from build123d import *

# Parameters (mm, degrees)
F0_W     = 60.565564
F0_H     = 97.339354
F1_DEPTH = 2.286
F2_R     = 2.032
F3_W     = 7.62
F3_H     = 3.81
F4_DEPTH = 0.127


with BuildPart() as f1:
    # F0 (on Front) → F1 (new body)
    with BuildSketch(Plane.XZ):
        Rectangle(F0_W, F0_H)
    extrude(amount=F1_DEPTH)

    # F2
    f2_edges = [f1.edges().sort_by_distance(p)[0] for p in [
        (30.282782, -2.286, 0),
        (-30.282782, -2.286, 0),
    ]]
    fillet(f2_edges, radius=F2_R)

    # F3 (on face) → F4 (join, symmetric)
    with BuildSketch(Plane(origin=(0, 0, 0), x_dir=(-1, 0, 0), z_dir=(0, 1, 0))):
        with Locations((-26.472782, -46.764677)):
            Rectangle(F3_W, F3_H)
        with Locations((26.472782, -46.764677)):
            Rectangle(F3_W, F3_H)
    extrude(amount=F4_DEPTH, both=True)


solid = f1.part
Could you check a few things on this model? Use its own coordinates, in mm. Give positions to 0.01 mm unless a question says otherwise; leave off trailing zeros. Write each loop counter-clockwise with the first axis right and the second up, starting at its lowest first coordinate (ties: lowest second). Pieces come first, ordered by that corner, then holes. Notation, with made-up numbers: (43, -15) - (99, -15) arc R22 cw to (99, 13) - close; hole circle Ø3 at (17, 23.5). An arc over 180 degrees is marked (long way). Use CSV: the item, a comma, the result in double quotes. Start each with the question number.
Item 1: I want a section at B-B, the plane x = -1. Please give me the cut outline in (y, z), then the cut area to 3 significant figures.
Item 2: I'm going to push a flat-ended pin straight in: pin 1 (18 mm diameter, centred on x = -14, z = -3.5, fed in from +Y). Where does the tip first touch, or does it pass through?
Item 3: If I drill on line 1 along Y through (x, z) = (18, -6.5); line 2 along X through (y, z) = (-0.35, -29); line 3 along X through (y, z) = (-1.7, -43), over which ranges is the centre line in solid material (lowest first)?
Item 4: I want a section at A-A, the plane z = 6. Please give me the cut outline in (x, y), then the cut area to 3 significant figures.
Item 5: I want a section at C-C, the plane y = -1.6. Please give me the cut outline in (x, z), then the cut area to 3 significant figures.
Findings:
1,outline,"(-2.29, -48.67) - (0, -48.67) - (0, 48.67) - (-2.29, 48.67) - close"
1,area,"223 mm2"
2,pin 1,"stops at y = 0"
3,line 1,"y = -2.29 to 0"
3,line 2,"x = -30.28 to 30.28"
3,line 3,"x = -29.68 to 29.68"
4,outline,"(-30.28, -0.25) arc R2.03 ccw to (-28.25, -2.29) - (28.25, -2.29) arc R2.03 ccw to (30.28, -0.25) - (30.28, 0) - (-30.28, 0) - close"
4,area,"137 mm2"
5,outline,"(-29.77, -48.67) - (29.77, -48.67) - (29.77, 48.67) - (-29.77, 48.67) - close"
5,area,"5,800 mm2"
